Work out the finished part from the listing and answer in its coordinate system (mm). A direction names the side the tool comes from. Round coordinates to 2 decimals unless told otherwise and drop trailing zeros. Write each loop counter-clockwise with the first axis right and the second up, starting at its lowest first coordinate (ties: lowest second). Pieces come first, ordered by that corner, then holes.
Autodesk Inventor part; units mm, degrees
ref_plane "YZ Plane" through (0, 0, 0) normal (1, 0, 0) x (0, 1, 0)
ref_plane "XZ Plane" through (0, 0, 0) normal (0, 1, 0) x (-1, 0, 0)
ref_plane "XY Plane" through (0, 0, 0) normal (0, 0, 1) x (1, 0, 0)
sketch "Szkic1" plane through (0, 0, 0) normal (0, 1, 0) x (-1, 0, 0)
  line L0 (0, 0) -> (97, 0)
  line L1 (97, 0) -> (97, -3)
  line L2 (97, -3) -> (0, -3)
  line L3 (0, -3) -> (0, 0)
  dimension "d0" = 97
  dimension "d1" = 3
extrude "Wyciągnięcie proste1" add sketch "Szkic1" along normal blind 8
sketch "Szkic2" plane through (0, 8, 0) normal (0, 1, 0) x (1, 0, 0)
  circle A0 centre (-94.6086, 1.3285) radius 1
  point P0 (0, 0)
  dimension "d4" = 2
extrude "Wyciągnięcie proste2" cut sketch "Szkic2" against normal blind 0.2
sketch "Szkic3" plane through (0, 0, -3) normal (0, 0, -1) x (-1, 0, 0)
  line L0 (0, 8) -> (97, 8)
  line L1 (0, 0) -> (3, 0)
  line L2 (3, 0) -> (3, 8)
  line L3 (3, 8) -> (0, 8)
  line L4 (0, 8) -> (0, 0)
  line L5 (0, 0) -> (97, 0)
  line L6 (97, 0) -> (94, 0)
  line L7 (94, 0) -> (94, 8)
  line L8 (94, 8) -> (97, 8)
  line L9 (97, 8) -> (97, 0)
  dimension "d7" = 3
  dimension "d8" = 3
extrude "Wyciągnięcie proste3" add sketch "Szkic3" along normal blind 19 contours L0 L2 L1 L4
extrude "Wyciągnięcie proste4" add sketch "Szkic3" along normal blind 20 contours L0 L9 L5 L7
sketch "Szkic4" plane through (-3, 0, -3) normal (-1, 0, 0) x (0, 0, 1)
  line L0 (-19, 0) -> (-19, 8)
  line L1 (0, 0) -> (-19, 0)
  line L2 (-19, 8) -> (-14, 8)
  line L3 (-14, 8) -> (-14, 0)
  line L4 (-14, 0) -> (-19, 0)
  line L5 (-19, 0) -> (-19, 8)
  point P0 (3, 0)
  dimension "d13" = 5
extrude "Wyciągnięcie proste5" add sketch "Szkic4" along normal blind 3
sketch "Szkic5" plane through (0, 8, 0) normal (0, 1, 0) x (1, 0, 0)
  line L0 (-3, 3) -> (-3, 17)
  line L1 (-3, 3) -> (-6, 3)
  line L2 (-6, 3) -> (-6, 6)
  line L3 (-6, 6) -> (-3, 6)
  line L4 (-3, 6) -> (-3, 3)
  point P0 (0, 0)
  dimension "d16" = 3
  dimension "d17" = 3
extrude "Wyciągnięcie proste6" add sketch "Szkic5" against normal blind 8
sketch "Szkic6" plane through (0, 8, 0) normal (0, 1, 0) x (1, 0, 0)
  line L0 (0, 0) -> (-6, 6)
  line L1 (-97, 0) -> (0, 0)
  line L2 (-6, 0) -> (0, 6)
  line L3 (0, 0) -> (0, 22)
  circle A0 centre (-3, 3) radius 2
  dimension "d20" = 4
extrude "Wyciągnięcie proste7" cut sketch "Szkic6" against normal blind 8 contours A0 L2 L0 | L0 L2 A0 | L2 A0 L0 | L0 A0 L2
sketch "Szkic7" plane through (0, 8, 0) normal (0, 1, 0) x (1, 0, 0)
  circle A0 centre (-3, 3) radius 2
  circle A1 centre (-3, 3) radius 2
  point P0 (0, 0)
extrude "Wyciągnięcie proste8" add sketch "Szkic7" against normal blind 3
sketch "Szkic8" plane through (0, 8, 0) normal (0, 1, 0) x (1, 0, 0)
  line L0 (-6, 3) -> (-94, 3)
  line L1 (-79, 3) -> (-73, 3)
  line L2 (-73, 3) -> (-73, 6)
  line L3 (-73, 6) -> (-79, 6)
  line L4 (-79, 6) -> (-79, 3)
  line L5 (-3, 6) -> (-3, 17)
  point P0 (0, 0)
  dimension "d25" = 6
  dimension "d26" = 3
  dimension "d27" = 70
extrude "Wyciągnięcie proste9" add sketch "Szkic8" against normal blind 8
sketch "Szkic9" plane through (0, 8, 0) normal (0, 1, 0) x (1, 0, 0)
  line L0 (-73, 3) -> (-73, 6)
  line L1 (-73, 6) -> (-78.8804, 0)
  line L2 (-97, 0) -> (0, 0)
  line L3 (-79, 3) -> (-79, 6)
  line L4 (-79, 6) -> (-72.878, 0)
  circle A0 centre (-75.939, 3) radius 2
  dimension "d30" = 4
extrude "Wyciągnięcie proste10" cut sketch "Szkic9" against normal blind 8 contours A0 L4 L1 | L1 L4 A0 | L4 A0 L1 | L1 A0 L4
sketch "Szkic10" plane through (0, 8, 0) normal (0, 1, 0) x (1, 0, 0)
  circle A0 centre (-75.939, 3) radius 2
  circle A1 centre (-75.939, 3) radius 2
  point P0 (0, 0)
extrude "Wyciągnięcie proste11" add sketch "Szkic10" against normal blind 3
sketch "Szkic11" plane through (-6, 0, -3) normal (0, 0, -1) x (-1, 0, 0)
  line L0 (67, 8) -> (67, 0)
  line L1 (91, 0) -> (-6, 0)
  line L2 (67, 8) -> (54, 8)
  line L3 (54, 8) -> (54, 0)
  line L4 (54, 0) -> (67, 0)
  line L5 (67, 0) -> (67, 8)
  dimension "d35" = 13
extrude "Wyciągnięcie proste12" cut sketch "Szkic11" against normal blind 0.5
sketch "Szkic13" plane through (-6, 0, -3) normal (0, 0, -1) x (-1, 0, 0)
  line L0 (54, 0) -> (54, 8)
  line L1 (0, 0) -> (0, 8)
  line L2 (54, 8) -> (0, 8)
  line L3 (0, 8) -> (0, 0)
  line L4 (0, 0) -> (54, 0)
  line L5 (54, 0) -> (54, 8)
  point P0 (-6, 0)
extrude "Wyciągnięcie proste14" cut sketch "Szkic13" against normal blind 0.75
sketch "Szkic14" plane through (-6, 0, -2.5) normal (0, 0, -1) x (-1, 0, 0)
  line L0 (67, 0) -> (54, 0)
  line L1 (67, 8) -> (67, 0)
  line L2 (54, 0) -> (67, 0)
  line L3 (67, 0) -> (67, 8)
  line L4 (67, 8) -> (54, 8)
  line L5 (54, 8) -> (54, 0)
  point P0 (-6, 0)
extrude "Wyciągnięcie proste15" cut sketch "Szkic14" against normal blind 0.25
sketch "Szkic15" plane through (-97, 0, 0) normal (-1, 0, 0) x (0, 0, 1)
  circle A0 centre (-19, 6) radius 1.5
  line L0 (-23, 0) -> (-23, 8)
  line L1 (0, 8) -> (-23, 8)
  point P0 (0, 0)
  dimension "d44" = 3
  dimension "d45" = 4
  dimension "d46" = 2
extrude "Wyciągnięcie proste16" cut sketch "Szkic15" against normal up to surface (3 mm away)
sketch "Szkic16" plane through (0, 0, 0) normal (0, -1, 0) x (1, 0, 0)
  line L0 (-3, -6) -> (-3, -17)
  line L1 (-6, -22) -> (-6, -17)
  line L2 (-3, -17) -> (-6, -17)
  line L3 (-6, -17) -> (-6, -22)
  line L4 (-6, -22) -> (-3, -22)
  line L5 (-3, -22) -> (-3, -17)
  point P0 (0, 0)
extrude "Wyciągnięcie proste17" cut sketch "Szkic16" against normal blind 8
sketch "Szkic17" plane through (0, 0, 0) normal (0, -1, 0) x (1, 0, 0)
  line L0 (0, 0) -> (0, -22)
  line L1 (0, -22) -> (-3, -22)
  line L2 (-3, -22) -> (-3, -19)
  line L3 (-3, -19) -> (0, -19)
  line L4 (0, -19) -> (0, -22)
  line L5 (0, -19) -> (-6, -19)
  line L6 (-6, -19) -> (-6, -25)
  line L7 (-6, -25) -> (0, -25)
  line L8 (0, -25) -> (0, -19)
  dimension "d51" = 3
  dimension "d52" = 3
  dimension "d53" = 6
  dimension "d54" = 6
extrude "Wyciągnięcie proste18" add sketch "Szkic17" against normal blind 3 contours L8 L7 L6 L5 L2 L1
sketch "Szkic18" plane through (0, 8, 0) normal (0, 1, 0) x (1, 0, 0)
  line L0 (0, 22) -> (-3, 22)
  line L1 (-3, 22) -> (-3, 19)
  line L2 (0, 22) -> (-3, 22)
  line L3 (-3, 22) -> (-3, 19)
  line L4 (-3, 19) -> (0, 19)
  line L5 (0, 19) -> (0, 22)
  point P0 (0, 0)
extrude "Wyciągnięcie proste19" cut sketch "Szkic18" against normal blind 5
sketch "Szkic19" plane through (0, 0, 0) normal (0, -1, 0) x (1, 0, 0)
  point P0 (0, 0)
sketch "Szkic20" plane through (0, 0, 0) normal (0, -1, 0) x (1, 0, 0)
  circle A0 centre (-3, -22) radius 2
  line L0 (-6, -25) -> (0, -25)
  line L1 (-6, -19) -> (-6, -25)
  point P0 (0, 0)
  point P1 (-6, -22)
  dimension "d59" = 4
  dimension "d60" = 3
  dimension "d61" = 3
extrude "Wyciągnięcie proste20" cut sketch "Szkic20" against normal blind 3
fillet "Fillet1" radius 3 2 edges at (-6, 1.5, -25) (-6, 1.5, -19)
fillet "Fillet2" radius 3 1 edges at (-6, 4, -6)
fillet "Zaokrąglenie3" radius 3 1 edges at (-73, 4, -6)
fillet "Zaokrąglenie4" radius 3 1 edges at (-79, 4, -6)
properties part number "lewasciana" material "Tworzywo sztuczne PET"
Q1. Find section A-A (z = -11.25). Determine the outline of the cut face in (x, y), plus the area to 3 significant figures.
Q2. Find section C-C (x = -36.5). Determine the outline of the cut face in (y, z).
Q3. Given pin 1 (2.5 mm diameter, centred on x = -3, z = -22, fed in from +Y); pin 2 (3.5 mm diameter, centred on x = -95.5, y = 6, fed in from -Z); pin 3 (3 mm diameter, centred on x = -4, z = -23, fed in from +Y), each flat-ended and moving along its own axis, determine where each tip first touches the part or whether it passes through.
Q4. A tool of negligible diameter and unlimited length cuts with its end or side. For faces 4 (the face through (-1, 3, -21)), 5 (the face through (-5.14, 1.52, -19.9)), 6 (the face through (-76, 5, -3)), from which of +Z, -Z, +X, -X, +Y, -Y can it reach the whole face along a straight path? Write none if from no direction.
Q5. Find the intervals of material crossed by L1, parallel to Z at x = -4, y = 1; L2, parallel to X at y = 7.5, z = -17.75; L3, parallel to X at y = 5.5, z = -4.25, in increasing order.
Q6. The mould has two halves that part along X. Classify faces 1 (the face through (-94, 4, -13)), 2 (the face through (-52, 8, -1)), 3 (the face through (-97, 4, -11)): +X half, -X half, draft (parallel to the pull), parting line (faces both ways), or undercut.
Report:
1. outline: (-97, 0) - (-94, 0) - (-94, 8) - (-97, 8) - close; (-3, 0) - (0, 0) - (0, 8) - (-3, 8) - close
1. area: 48.0 mm2
2. outline: (0, -2.25) - (8, -2.25) - (8, 0) - (0, 0) - close
3. pin 1: passes through
3. pin 2: stops at z = -23
3. pin 3: stops at y = 3
4. face 4: -Z, +X, +Y
4. face 5: +Y, -Y
4. face 6: -Y
5. L1: z = -24.83 to -23.73, -20.27 to -19.17, -5.83 to -4.73, -1.27 to 0
5. L2: x = -97 to -94, -3 to 0
5. L3: x = -97 to -94, -78.73 to -73.27, -5.73 to 0
6. face 1: undercut
6. face 2: draft
6. face 3: -X half
